Geometry check sheet. Reference: the model listing, model coordinates, mm. Face numbers are marked on the shaded views. A direction names the side the tool comes from. Coordinates: 2 decimals unless noted, no trailing zeros. Order: outer loops, then holes, each group sorted by start corner. A loop starts at its lowest first (then second) coordinate and runs counter-clockwise, first axis right, second up. Notation, with made-up numbers: M -19,70 L 37,70 A26 cw 37,91 Z; hole C -4.75,61 d4. An arc over 180 degrees is marked long. One line per item, written item: value. Start each with the question number.
1) Go/stop test with flat-tipped pins: P1, Ø5.5, axis at x = 26.5, z = -21, coming from the -Y side; P2, Ø11.5, axis at x = 41, z = -21.5, coming from the -Y side; P3, Ø3, axis at x = -24, z = -30.5, coming from the +Y side. Record where each tip stops, or that it passes through.
2) Sectioned sample at C-C, the plane z = -2.5. Enter the section's corners in (x, y).
3) Draft check along Z on the marked faces 6, 7 and 8. Enter one of: pulls with the +Z half, pulls with the -Z half, needs draft (parallel to the pull), parting line crosses it, or undercut.
4) Sectioned sample at A-A, the plane y = 2. Enter the section's corners in (x, z) (3 decimals).
5) Sectioned sample at B-B, the plane x = -9.5. Enter the section's corners in (y, z), then the cut area to 3 significant figures.
6) Sectioned sample at D-D, the plane x = 24. Enter the section's corners in (y, z), then the cut area to 3 significant figures.
7) Thickness scan on L1, parallel to Z at x = 15, y = 8.5; L2, parallel to X at y = 3, z = 50.5; L3, parallel to X at y = 12, z = 31.5. Record the ranges inside material, lowest first. Write a range as from..to.
8) Access from +Z, -Z, +X, -X, +Y, -Y to the whole of each face (thin tool, end or side, straight path). Record for the marked faces 1, 2, 3, 4 and 5.
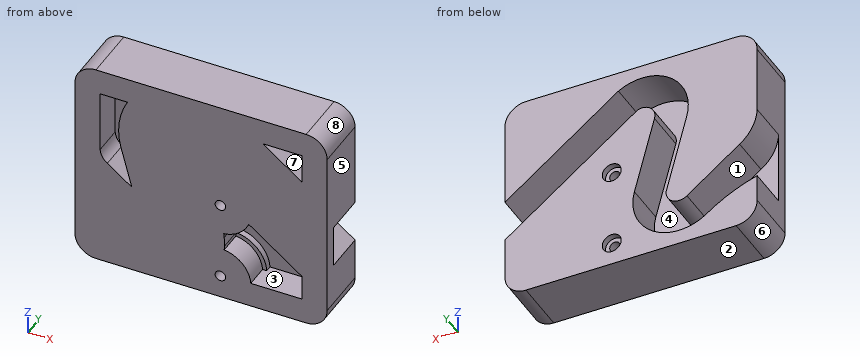
```python
from build123d import *

# Parameters (mm, degrees)
BOSS_EXTRUDE1_DEPTH = 33.02
CUT_EXTRUDE1_DEPTH  = 25.4
SKETCH3_R           = 3.175
CUT_EXTRUDE2_DEPTH  = 113.70847528
SKETCH4_R           = 5.715
SKETCH4_R_2         = 3.175
CUT_EXTRUDE3_DEPTH  = 3.81
SHELL4_DEPTH        = 17.78
SHELL4_2_DEPTH      = 13.97


# Read off the part's stored shape, not the designer's step: Shell4
with BuildPart() as part:
    # Sketch1 → Boss-Extrude1 (new body)
    with BuildSketch(Plane(origin=(0, 0, 0), x_dir=(1, 0, 0), z_dir=(0, 1, 0))):
        with BuildLine():
            Line((-63.5, -76.2), (63.5, -76.2))
            ThreePointArc((63.5, -76.2), (72.480256121, -72.480256121), (76.2, -63.5))
            Line((76.2, -63.5), (76.2, 38.1))
            ThreePointArc((76.2, 38.1), (72.480256121, 47.080256121), (63.5, 50.8))
            Line((63.5, 50.8), (-63.5, 50.8))
            ThreePointArc((-63.5, 50.8), (-72.480256121, 47.080256121), (-76.2, 38.1))
            Line((-76.2, 38.1), (-76.2, -63.5))
            ThreePointArc((-76.2, -63.5), (-72.480256121, -72.480256121), (-63.5, -76.2))
        make_face()
    extrude(amount=BOSS_EXTRUDE1_DEPTH)

    # Sketch2 → Cut-Extrude1 (cut)
    with BuildSketch(Plane(origin=(0, 33.02, 0), x_dir=(1, 0, 0), z_dir=(0, 1, 0))):
        with BuildLine():
            Line((-21.234187682, 13.253251383), (-33.621595815, -32.977185142))
            ThreePointArc((-33.621595815, -32.977185142), (-23.484698626, -62.452913285), (7.640823288, -64.119382534))
            Line((7.640823288, -64.119382534), (76.2, -12.7))
            Line((76.2, -12.7), (76.2, 12.7))
            Line((76.2, 12.7), (-3.941576712, -47.406182534))
            ThreePointArc((-3.941576712, -47.406182534), (-11.856979187, -45.921156496), (-14.138642435, -38.197626766))
            Line((-14.138642435, -38.197626766), (-2.029571171, 6.994042425))
            ThreePointArc((-2.029571171, 6.994042425), (-13.371601822, 37.382259223), (-45.797751473, 36.588408962))
            ThreePointArc((-45.797751473, 36.588408962), (-60.308353779, 27.645114035), (-76.2, 21.481050133))
            Line((-76.2, 21.481050133), (-76.2, -23.043277433))
            ThreePointArc((-76.2, -23.043277433), (-73.166835121, -11.965986434), (-65.564641264, -3.357089081))
            Line((-65.564641264, -3.357089081), (-33.739992737, 20.511397314))
            ThreePointArc((-33.739992737, 20.511397314), (-25.085058678, 21.02103117), (-21.234187682, 13.253251383))
        make_face()
    extrude(amount=-CUT_EXTRUDE1_DEPTH, mode=Mode.SUBTRACT)

    # Sketch3 → Cut-Extrude2 (cut, through all)
    with BuildSketch(Plane(origin=(0, 33.02, 0), x_dir=(1, 0, 0), z_dir=(0, 1, 0))):
        with Locations(Location((11.674814186, 36.83, 0), (0, 0, 270))):
            Circle(SKETCH3_R)
        with Locations(Location((11.674814186, -10.616391667, 0), (0, 0, 270))):
            Circle(SKETCH3_R)
    extrude(amount=-CUT_EXTRUDE2_DEPTH, mode=Mode.SUBTRACT)

    # Sketch4 → Cut-Extrude3 (cut)
    # profile 1 of 2: a face of its own
    with BuildSketch(Plane(origin=(0, 33.02, 0), x_dir=(1, 0, 0), z_dir=(0, 1, 0))):
        with Locations(Location((11.674814186, 36.83, 0), (0, 0, 270))):
            Circle(SKETCH4_R)
    # profile 2 of 2: a face of its own
    with BuildSketch(Plane(origin=(0, 33.02, 0), x_dir=(1, 0, 0), z_dir=(0, 1, 0))):
        with Locations(Location((11.674814186, -10.616391667, 0), (0, 0, 270))):
            Circle(SKETCH4_R)
        with Locations(Location((11.674814186, -10.616391667, 0), (0, 0, 270))):
            Circle(SKETCH4_R_2, mode=Mode.SUBTRACT)
    extrude(amount=-CUT_EXTRUDE3_DEPTH, mode=Mode.SUBTRACT)

    # Shell4 outline → Shell4 (cut)
    with BuildSketch(Plane(origin=(0, 0, 0), x_dir=(1, 0, 0), z_dir=(0, 1, 0))):
        with BuildLine():
            Line((-41.788947679, -4.575318892), (-56.600935015, -15.684309395))
            ThreePointArc((-56.600935015, -15.684309395), (-59.668026883, -19.046046541), (-60.96, -23.409432225))
            Line((-60.96, -23.409432225), (-60.96, -60.96))
            Line((-60.96, -60.96), (-44.483340176, -60.96))
            ThreePointArc((-44.483340176, -60.96), (-49.500189899, -45.369554015), (-48.342305407, -29.032782895))
            Line((-48.342305407, -29.032782895), (-41.788947679, -4.575318892))
        make_face()
        Polygon((37.253333333, -60.96), (60.96, -60.96), (60.96, -43.18), align=None)
        with BuildLine():
            ThreePointArc((13.975676971, 10.211907722), (24.100715908, 6.256930217), (30.882136703, -2.238397473))
            Line((30.882136703, -2.238397473), (60.96, 20.32))
            Line((60.96, 20.32), (60.96, 35.56))
            Line((60.96, 35.56), (32.591293933, 35.56))
            ThreePointArc((32.591293933, 35.56), (26.905461548, 22.437661554), (14.125676613, 16.018817949))
            ThreePointArc((14.125676613, 16.018817949), (14.148411798, 13.11283822), (13.975676971, 10.211907722))
        make_face()
    extrude(amount=SHELL4_DEPTH, mode=Mode.SUBTRACT)

    # Shell4 2 outline → Shell4 2 (cut)
    with BuildSketch(Plane(origin=(0, 0, 0), x_dir=(1, 0, 0), z_dir=(0, 1, 0))):
        with BuildLine():
            Line((28.785986128, -3.810510404), (30.882136703, -2.238397473))
            ThreePointArc((30.882136703, -2.238397473), (24.100715908, 6.256930217), (13.975676971, 10.211907722))
            ThreePointArc((13.975676971, 10.211907722), (13.838972267, 8.949034749), (13.66518896, 7.690728075))
            ThreePointArc((13.66518896, 7.690728075), (22.823217362, 4.040529279), (28.785986128, -3.810510404))
        make_face()
        with BuildLine():
            ThreePointArc((13.945477939, 18.555528431), (14.054251914, 17.288499768), (14.125676613, 16.018817949))
            ThreePointArc((14.125676613, 16.018817949), (26.905461548, 22.437661554), (32.591293933, 35.56))
            Line((32.591293933, 35.56), (30.045968886, 35.56))
            ThreePointArc((30.045968886, 35.56), (25.046769189, 24.168916144), (13.945477939, 18.555528431))
        make_face()
    extrude(amount=SHELL4_2_DEPTH, mode=Mode.SUBTRACT)


solid = part.part
```
Final values:
1. P1: stops at y = 13.97
1. P2: stops at y = 17.78
1. P3: stops at y = 7.62
2. outline: M -76.2,0 L 24.6,0 L 24.6,13.97 L 28.02,13.97 L 28.02,17.78 L 37.2,17.78 L 37.2,0 L 76.2,0 L 76.2,7.62 L 62.6,7.62 L 62.6,33.02 L -3.23,33.02 L -3.23,7.62 L -24.12,7.62 L -24.12,33.02 L -57.76,33.02 L -57.76,7.62 L -76.2,7.62 Z
3. face 6: pulls with the -Z half
3. face 7: undercut
3. face 8: pulls with the +Z half
4. outline: M -76.2,-38.1 A12.7 ccw -63.5,-50.8 L 63.5,-50.8 A12.7 ccw 76.2,-38.1 L 76.2,63.5 A12.7 ccw 63.5,76.2 L -63.5,76.2 A12.7 ccw -76.2,63.5 Z; hole M -60.96,23.409 A10.16 ccw -56.601,15.684 L -41.789,4.575 L -48.342,29.033 A43.126 cw -44.483,60.96 L -60.96,60.96 Z; hole C 11.675,-36.83 d6.35; hole C 11.675,10.616 d6.35; hole M 13.665,-7.691 A43.19 cw 13.976,-10.212 A43.19 cw 14.126,-16.019 A43.19 cw 13.945,-18.556 A18.415 cw 30.046,-35.56 L 60.96,-35.56 L 60.96,-20.32 L 28.786,3.811 A18.415 cw Z; hole M 37.253,60.96 L 60.96,43.18 L 60.96,60.96 Z
5. outline: M 0,-50.8 L 33.02,-50.8 L 33.02,-34.23 L 7.62,-34.23 L 7.62,20.89 L 33.02,20.89 L 33.02,47.38 L 7.62,47.38 L 7.62,67.94 L 33.02,67.94 L 33.02,76.2 L 0,76.2 Z
5. area: 2,270 mm^2
6. outline: M 0,-50.8 L 33.02,-50.8 L 33.02,26.45 L 7.62,26.45 L 7.62,51.85 L 33.02,51.85 L 33.02,76.2 L 0,76.2 L 0,-3.07 L 13.97,-3.07 L 13.97,-6.33 L 17.78,-6.33 L 17.78,-19.88 L 13.97,-19.88 L 13.97,-23.15 L 0,-23.15 Z
6. area: 3,220 mm^2
7. L1: z = -50.8..-18.72, -7.5..33.2, 58.6..76.2
7. L2: x = -76.2..-60.96, -48.56..51.2, 60.96..76.2
7. L3: x = -76.2..-60.96, -48.93..-33.23, -12.34..17.27, 51.13..76.2
8. face 1: -X, +Y
8. face 2: -Z, +X, -X, +Y, -Y
8. face 3: -Y
8. face 4: +Y
8. face 5: +Z, -Z, +X, +Y, -Y
